Input: part model. Units: mm. Frame: model coordinates. A direction names the side the tool comes from. Coordinates: 2 decimals unless noted, no trailing zeros. Loops run counter-clockwise (first coordinate to the right, second up) from the corner with the lowest first, then second, coordinate; pieces in that order, holes last.
Item 1: Contact query for flat-ended pins moving along their axis: P1, Ø9.5, axis at y = -6, z = -11.6, coming from the -X side; P2, Ø5, axis at y = 24, z = 17.5, coming from the +X side; P3, Ø6.5, axis at x = 19, y = -37, coming from the -Z side (3 decimals). Output: stop coordinate, or through.
Item 2: Section A-A on z = 77.6. Return loops of the section in (x, y) (3 decimals).
Item 3: Section D-D on x = 18. Return loops of the section in (y, z) (3 decimals).
Item 4: Pull-direction query (Z, two-part tool) for faces 5 (the cylindrical face through (52.42, 8.38, 21.58)), 6 (the flat face through (11, 62, 36)), 7 (the flat face through (15, 31, 146)); classes: released by +Z, released by -Z, zero draft, split by the parting line, or undercut.
Item 5: Reachability of faces 1 (the flat face through (46.5, -9, 42)), 2 (the flat face through (18, -38, 31.225)), 3 (the flat face through (9.56, 47, 35)), 4 (the flat face through (5, 6, 73)) from +Z, -Z, +X, -X, +Y, -Y: full face, straight path, thin tool, end or side. Return the list, or none.
Item 6: Section B-B on x = 25.5. Return loops of the section in (y, z).
Item 7: Ray query, line 1 along X through (y, z) = (-2.5, 14.5); line 2 along Y through (x, z) = (16.5, 21.7) (3 decimals); line 3 along Y through (x, z) = (17, 33). Return the intervals inside material, ascending.
Item 8: Section C-C on y = 37. Return loops of the section in (x, z).
```python
from build123d import *

# Parameters (mm, degrees)
SKETCH1_R                       = 33
BOSS_EXTRUDE1_DEPTH             = 21.5
SKETCH4_R                       = 20
BOSS_EXTRUDE4_DEPTH             = 37
SKETCH6_W                       = 21.5
SKETCH6_H                       = 62
BOSS_EXTRUDE5_DEPTH             = 73
BOSS_EXTRUDE6_DEPTH             = 73
BOSS_EXTRUDE7_DEPTH             = 8
M6X1_0_TAPPED_HOLE1_D           = 5
M6X1_0_TAPPED_HOLE1_DEPTH       = 14.99
M6X1_0_TAPPED_HOLE1_CBORE_D     = 6
M6X1_0_TAPPED_HOLE1_CBORE_DEPTH = 11.94
M6X1_0_TAPPED_HOLE1_TIP         = 1.502151548
M5X0_8_TAPPED_HOLE1_D           = 4.2
M5X0_8_TAPPED_HOLE1_DEPTH       = 12.192
M5X0_8_TAPPED_HOLE1_TIP         = 1.2618073
SKETCH14_W                      = 25
SKETCH14_H                      = 8


with BuildPart() as part:
    # Sketch1 → Boss-Extrude1 (new body)
    with BuildSketch(Plane(origin=(0, 0, 0), x_dir=(0, 0, -1), z_dir=(1, 0, 0))):
        with Locations((-33, 0)):
            Circle(SKETCH1_R)
    extrude(amount=BOSS_EXTRUDE1_DEPTH)

    # Sketch4 → Boss-Extrude4 (add)
    with BuildSketch(Plane(origin=(21.5, 0, 0), x_dir=(0, 0, -1), z_dir=(1, 0, 0))):
        with Locations((-33, 0)):
            Circle(SKETCH4_R)
    extrude(amount=BOSS_EXTRUDE4_DEPTH)

    # Sketch6 → Boss-Extrude5 (add)
    with BuildSketch(Plane.XY):
        with Locations((10.75, 31)):
            Rectangle(SKETCH6_W, SKETCH6_H)
    extrude(amount=BOSS_EXTRUDE5_DEPTH)

    # Sketch7 → Boss-Extrude6 (add)
    with BuildSketch(Plane.XY.offset(73)):
        with BuildLine():
            Line((30.3, 41), (30.3, 21))
            ThreePointArc((30.3, 21), (15.15, 5.85), (0, 21))
            Line((0, 21), (0, 41))
            ThreePointArc((0, 41), (15.15, 56.15), (30.3, 41))
        make_face()
    extrude(amount=BOSS_EXTRUDE6_DEPTH)

    # Sketch9 → Boss-Extrude7 (add)
    with BuildSketch(Plane(origin=(21.5, 0, 0), x_dir=(0, 0, -1), z_dir=(1, 0, 0))):
        with BuildLine():
            Line((11.6, 3.525), (0, 3.525))
            Line((0, 3.525), (-3.880000429, -15.525))
            Line((-3.880000429, -15.525), (11.6, -15.525))
            ThreePointArc((11.6, -15.525), (21.125, -6), (11.6, 3.525))
        make_face()
        with BuildLine():
            Line((-12.175, -43.5), (-12.175, -25.599206531))
            Line((-12.175, -25.599206531), (-31.225, -32.95222868))
            Line((-31.225, -32.95222868), (-31.225, -43.5))
            ThreePointArc((-31.225, -43.5), (-21.7, -53.025), (-12.175, -43.5))
        make_face()
        with BuildLine():
            Line((-82.269569588, 2.301851893), (-73, 7.245000909))
            Line((-73, 7.245000909), (-63.910592017, 7.245000909))
            Line((-63.910592017, 7.245000909), (-63.910592017, -11.555747537))
            Line((-63.910592017, -11.555747537), (-74.647866464, -15.055966684))
            ThreePointArc((-74.647866464, -15.055966684), (-86.321287926, -9.829459741), (-82.269569588, 2.301851893))
        make_face()
    extrude(amount=-BOSS_EXTRUDE7_DEPTH)

    # M6x1.0 Tapped Hole1
    with Locations(Plane(origin=(21.5, 0, 0), x_dir=(0, 0, -1), z_dir=(1, 0, 0))):
        with Locations((-33, 45), (11.6, -6), (-21.7, -43.5), (-77.6, -6)):
            CounterBoreHole(M6X1_0_TAPPED_HOLE1_D / 2, M6X1_0_TAPPED_HOLE1_CBORE_D / 2, M6X1_0_TAPPED_HOLE1_CBORE_DEPTH, depth=M6X1_0_TAPPED_HOLE1_DEPTH)
            with Locations((0, 0, -(M6X1_0_TAPPED_HOLE1_DEPTH + M6X1_0_TAPPED_HOLE1_TIP / 2))):  # 118° drill point
                Cone(0, M6X1_0_TAPPED_HOLE1_D / 2, M6X1_0_TAPPED_HOLE1_TIP, mode=Mode.SUBTRACT)

    # M5x0.8 Tapped Hole1
    with Locations(Plane(origin=(58.5, 0, 0), x_dir=(0, 0, -1), z_dir=(1, 0, 0))):
        with Locations((-19.576606241, 7.75), (-33, -15.5), (-46.423393759, 7.75)):
            Hole(M5X0_8_TAPPED_HOLE1_D / 2, depth=M5X0_8_TAPPED_HOLE1_DEPTH)
            with Locations((0, 0, -(M5X0_8_TAPPED_HOLE1_DEPTH + M5X0_8_TAPPED_HOLE1_TIP / 2))):  # 118° drill point
                Cone(0, M5X0_8_TAPPED_HOLE1_D / 2, M5X0_8_TAPPED_HOLE1_TIP, mode=Mode.SUBTRACT)

    # Sketch14 → Cut-Revolve1 (revolve, cut)
    with BuildSketch(Plane(origin=(0, 0, 0), x_dir=(1, 0, 0), z_dir=(0, 1, 0))):
        with Locations((34, -49)):
            Rectangle(SKETCH14_W, SKETCH14_H)
    revolve(axis=Axis((58.5, 0, 33), (-1, 0, 0)), mode=Mode.SUBTRACT)


solid = part.part
```
Results found:
1. P1: stops at x = 13.5
1. P2: stops at x = 21.5
1. P3: stops at z = 12.175
2. outline: (0, 21) arc R15.15 ccw to (30.3, 21) - (30.3, 41) arc R15.15 ccw to (0, 41) - close; (13.5, -15.525) - (21.5, -15.525) - (21.5, -9) - (13.5, -9) - close; (13.5, -3) - (21.5, -3) - (21.5, 4.792) - (13.5, 4.792) - close
3. outline: (-43.5, 12.175) - (-25.599, 12.175) arc R33 ccw to (-15.525, 3.88) - (-15.525, -11.6) arc R9.525 ccw to (3.525, -11.6) - (3.525, 0) - (62, 0) - (62, 73) - (55.88, 73) - (55.88, 146) - (6.12, 146) - (6.12, 75.109) - (2.302, 82.27) arc R9.525 ccw to (-15.056, 74.648) - (-11.556, 63.911) arc R33 ccw to (-32.952, 31.225) - (-43.5, 31.225) arc R9.525 ccw to start; hole circle Ø6 at (-43.5, 21.7); hole circle Ø6 at (-6, -11.6); hole circle Ø6 at (-6, 77.6); hole circle Ø6 at (45, 33)
4. face 5: undercut
4. face 6: zero draft
4. face 7: released by +Z
5. face 1: none
5. face 2: +Z, +X, -X, -Y
5. face 3: +X
5. face 4: +Z, -X, -Y
6. outline: circle Ø24 at (0, 33); (9.94, 73) - (52.06, 73) - (52.06, 146) - (9.94, 146) - close
7. line 1: x = 0 to 21.5, 46.5 to 58.5
7. line 2: y = -53.025 to -46.5, -40.5 to 62
7. line 3: y = -33 to 42, 48 to 62
8. outline: (0, 0) - (21.5, 0) - (21.5, 73) - (30.3, 73) - (30.3, 146) - (0, 146) - close
